```python
from build123d import *

# Parameters (mm, degrees)
SKETCH1_W           = 10
SKETCH1_H           = 8
BOSS_EXTRUDE1_DEPTH = 5
SKETCH2_W           = 9.8
SKETCH2_H           = 1.3
BOSS_EXTRUDE2_DEPTH = 6
SKETCH3_W           = 6.3
SKETCH3_H           = 0.5
BOSS_EXTRUDE3_DEPTH = 2.5
BOSS_EXTRUDE4_START = -6.3
BOSS_EXTRUDE4_DEPTH = 6.3
SKETCH5_W           = 1.2
SKETCH5_H           = 5
CUT_EXTRUDE1_DEPTH  = 14.190905958
SKETCH6_W           = 0.275
SKETCH6_H           = 5
SKETCH6_W_2         = 0.2
CUT_EXTRUDE2_DEPTH  = 3.5
SKETCH7_R           = 1.8
CUT_EXTRUDE3_DEPTH  = 3.5
SKETCH8_W           = 0.11872329
SKETCH8_H           = 1.322916667
CUT_EXTRUDE4_DEPTH  = 3.5


with BuildPart() as part:
    # Sketch1 → Boss-Extrude1 (new body)
    with BuildSketch(Plane(origin=(0, 0, 0), x_dir=(1, 0, 0), z_dir=(0, 1, 0))):
        Rectangle(SKETCH1_W, SKETCH1_H)
    extrude(amount=BOSS_EXTRUDE1_DEPTH)

    # Sketch2 → Boss-Extrude2 (add)
    with BuildSketch(Plane(origin=(0, 0, -4), x_dir=(-1, 0, 0), z_dir=(0, 0, -1))):
        with Locations((0, 0.65)):
            Rectangle(SKETCH2_W, SKETCH2_H)
    extrude(amount=BOSS_EXTRUDE2_DEPTH)

    # Sketch3 → Boss-Extrude3 (add)
    with BuildSketch(Plane.XY.offset(4)):
        with Locations((0, 3.75)):
            Rectangle(SKETCH3_W, SKETCH3_H)
    extrude(amount=BOSS_EXTRUDE3_DEPTH)

    # Sketch4 → Boss-Extrude4 (add)
    with BuildSketch(Plane.ZY.offset(3.15).offset(BOSS_EXTRUDE4_START)):
        with BuildLine():
            Line((7.714456463, 2), (7.714456463, -3))
            Line((7.714456463, -3), (8.214456463, -3))
            Line((8.214456463, -3), (8.214456463, 2))
            ThreePointArc((8.214456463, 2), (7.756212161, 3.342020289), (6.5, 4))
            Line((6.5, 4), (6.5, 3.5))
            ThreePointArc((6.5, 3.5), (7.40002744, 2.98706126), (7.714456463, 2))
        make_face()
    extrude(amount=BOSS_EXTRUDE4_DEPTH)

    # Sketch5 → Cut-Extrude1 (cut, through all)
    with BuildSketch(Plane(origin=(0, 4, 0), x_dir=(1, 0, 0), z_dir=(0, 1, 0))):
        with Locations((-1.2, -6.5)):
            Rectangle(SKETCH5_W, SKETCH5_H)
        with Locations((1.2, -6.5)):
            Rectangle(SKETCH5_W, SKETCH5_H)
    extrude(amount=-CUT_EXTRUDE1_DEPTH, mode=Mode.SUBTRACT)

    # Sketch6 → Cut-Extrude2 (cut)
    with BuildSketch(Plane.XY.offset(8.214456463)):
        with Locations((-3.0125, -0.5)):
            Rectangle(SKETCH6_W, SKETCH6_H)
        with Locations((-1.9375, -0.5)):
            Rectangle(SKETCH6_W, SKETCH6_H)
        with Locations((-0.5, -0.5)):
            Rectangle(SKETCH6_W_2, SKETCH6_H)
        with Locations((0.5, -0.5)):
            Rectangle(SKETCH6_W_2, SKETCH6_H)
        with Locations((1.9375, -0.5)):
            Rectangle(SKETCH6_W, SKETCH6_H)
        with Locations((3.0125, -0.5)):
            Rectangle(SKETCH6_W, SKETCH6_H)
    extrude(amount=-CUT_EXTRUDE2_DEPTH, mode=Mode.SUBTRACT)

    # Sketch7 → Cut-Extrude3 (cut)
    with BuildSketch(Plane(origin=(0, 1.3, 0), x_dir=(1, 0, 0), z_dir=(0, 1, 0))):
        with Locations(Location((0, 8, 0), (0, 0, 270))):
            Circle(SKETCH7_R)
    extrude(amount=-CUT_EXTRUDE3_DEPTH, mode=Mode.SUBTRACT)

    # Sketch8 → Cut-Extrude4 (cut)
    # profile 1 of 7: a face of its own
    with BuildSketch(Plane(origin=(0, 5, 0), x_dir=(1, 0, 0), z_dir=(0, 1, 0))):
        with Locations((-3.24297038, 1.408129396)):
            Rectangle(SKETCH8_W, SKETCH8_H)
    # profile 2 of 7: a face of its own
    with BuildSketch(Plane(origin=(0, 5, 0), x_dir=(1, 0, 0), z_dir=(0, 1, 0))):
        with BuildLine():
            Line((-2.844399333, 2.069587729), (-2.579656995, 2.069587729))
            add(Edge.make_bspline(
                [(-2.579656995, 2.069587729), (-2.561989961, 2.069528921), (-2.5280673, 2.069416003), (-2.479469665, 2.068786385), (-2.435311804, 2.066981792), (-2.395616805, 2.065428845), (-2.360385397, 2.06259707), (-2.329509546, 2.059890516), (-2.303131458, 2.056347495), (-2.287163532, 2.053057052), (-2.279933688, 2.051567229)],
                knots=[0, 0, 0, 0, 1.410062039, 2.707475311, 3.878576406, 4.937260626, 5.877586885, 6.699081471, 7.410979367, 8, 8, 8, 8], degree=3))
            add(Edge.make_bspline(
                [(-2.279933688, 2.051567229), (-2.270254994, 2.049175863), (-2.251104078, 2.044444144), (-2.22353069, 2.034443045), (-2.19725593, 2.022869555), (-2.172388943, 2.009276125), (-2.149054284, 1.993561849), (-2.127011351, 1.975998005), (-2.106160119, 1.956680698), (-2.087343849, 1.935122886), (-2.069602005, 1.91250611), (-2.054638446, 1.88804963), (-2.04173945, 1.862475184), (-2.031469641, 1.835522678), (-2.023200288, 1.807453496), (-2.017369537, 1.778013385), (-2.013872808, 1.747336469), (-2.013516809, 1.726412498), (-2.013336299, 1.715802923)],
                knots=[0, 0, 0, 0, 1.027469482, 2.033020251, 3.019912614, 3.986113645, 4.951240523, 5.91722682, 6.890402269, 7.87763091, 8.8651537, 9.85103654, 10.82876324, 11.815024772, 12.821070561, 13.842952187, 14.906261191, 16, 16, 16, 16], degree=3))
            add(Edge.make_bspline(
                [(-2.013336299, 1.715802923), (-2.013891545, 1.698175964), (-2.014974974, 1.663781201), (-2.025076427, 1.613865332), (-2.041622909, 1.567302704), (-2.064423676, 1.524151945), (-2.093459609, 1.485254172), (-2.128356182, 1.451088732), (-2.169132862, 1.422498646), (-2.207092753, 1.402672734), (-2.240624608, 1.389975415), (-2.268229461, 1.381041434), (-2.298341682, 1.374138846), (-2.330672758, 1.367955106), (-2.365357235, 1.363286459), (-2.402311982, 1.359867062), (-2.441563355, 1.357729966), (-2.468527824, 1.357411708), (-2.482399299, 1.357247985)],
                knots=[0, 0, 0, 0, 1.260483769, 2.459530307, 3.627416485, 4.787058657, 5.939039949, 7.08810263, 8.267026773, 9.491475466, 10.141966685, 10.831826277, 11.566392101, 12.351337768, 13.187381173, 14.07005841, 15.007169909, 16, 16, 16, 16], degree=3))
            Line((-2.482399299, 1.357247985), (-1.996375829, 0.746671062))
            Line((-1.996375829, 0.746671062), (-2.143189898, 0.746671062))
            Line((-2.143189898, 0.746671062), (-2.629213369, 1.357247985))
            Line((-2.629213369, 1.357247985), (-2.725676042, 1.357247985))
            Line((-2.725676042, 1.357247985), (-2.725676042, 0.746671062))
            Line((-2.725676042, 0.746671062), (-2.844399333, 0.746671062))
            Line((-2.844399333, 0.746671062), (-2.844399333, 2.069587729))
        make_face()
        with BuildLine():
            Line((-2.725676042, 1.933903968), (-2.725676042, 1.492931746))
            Line((-2.725676042, 1.492931746), (-2.483459329, 1.491076694))
            add(Edge.make_bspline(
                [(-2.483459329, 1.491076694), (-2.472150266, 1.491071691), (-2.450230083, 1.491061994), (-2.418517629, 1.492571546), (-2.388990087, 1.494288812), (-2.361760398, 1.496915499), (-2.336816398, 1.500300681), (-2.314170554, 1.504535143), (-2.2937859, 1.509468511), (-2.27001175, 1.517104245), (-2.243464014, 1.529201758), (-2.214612539, 1.546802408), (-2.190043203, 1.56894014), (-2.169285559, 1.594254512), (-2.152605685, 1.622087261), (-2.140846069, 1.652104758), (-2.133383896, 1.683549201), (-2.132503761, 1.705161164), (-2.132059589, 1.71606793)],
                knots=[0, 0, 0, 0, 1.146690395, 2.22261258, 3.21895312, 4.145990853, 4.996080663, 5.770904154, 6.481378293, 7.121626537, 8.300444488, 9.431385265, 10.535395872, 11.636531494, 12.74115979, 13.810798291, 14.895190096, 16, 16, 16, 16], degree=3))
            add(Edge.make_bspline(
                [(-2.132059589, 1.71606793), (-2.132513962, 1.726706665), (-2.133414364, 1.747788755), (-2.140765536, 1.778652745), (-2.153196939, 1.807782217), (-2.169949689, 1.835058675), (-2.190360084, 1.859818283), (-2.21429271, 1.881002772), (-2.241093185, 1.898483969), (-2.26614212, 1.909654821), (-2.288531242, 1.916503694), (-2.307970429, 1.921323331), (-2.329935184, 1.925195496), (-2.354532158, 1.928297947), (-2.381656346, 1.930964548), (-2.411444896, 1.932760608), (-2.443700167, 1.933824181), (-2.466056299, 1.933876754), (-2.477629167, 1.933903968)],
                knots=[0, 0, 0, 0, 1.101028733, 2.181837193, 3.264309656, 4.369019818, 5.486613113, 6.575447106, 7.666700264, 8.788928104, 9.402425223, 10.0903467, 10.862060571, 11.710948788, 12.657782767, 13.684531032, 14.801375019, 16, 16, 16, 16], degree=3))
            Line((-2.477629167, 1.933903968), (-2.725676042, 1.933903968))
        make_face(mode=Mode.SUBTRACT)
    # profile 3 of 7: a face of its own
    with BuildSketch(Plane(origin=(0, 5, 0), x_dir=(1, 0, 0), z_dir=(0, 1, 0))):
        Polygon((-1.725008307, 2.069587729), (-1.606285017, 2.069587729), (-1.606285017, 0.882354823), (-1.097470914, 0.882354823), (-1.097470914, 0.746671062), (-1.725008307, 0.746671062), align=None)
    # profile 4 of 7: a face of its own
    with BuildSketch(Plane(origin=(0, 5, 0), x_dir=(1, 0, 0), z_dir=(0, 1, 0))):
        Polygon((-0.944826683, 1.933903968), (-0.944826683, 2.069587729), (-0.24944741, 2.069587729), (-0.80437279, 0.882354823), (-0.26640788, 0.882354823), (-0.26640788, 0.746671062), (-0.995708093, 0.746671062), (-0.440782713, 1.933903968), align=None)
    # profile 5 of 7: a face of its own
    with BuildSketch(Plane(origin=(0, 5, 0), x_dir=(1, 0, 0), z_dir=(0, 1, 0))):
        Polygon((0.608381366, 2.103508669), (0.632497035, 2.103508669), (0.632497035, 1.187643284), (0.785141265, 1.187643284), (0.785141265, 1.051959524), (0.632497035, 1.051959524), (0.632497035, 0.746671062), (0.513773744, 0.746671062), (0.513773744, 1.051959524), (-0.113763649, 1.051959524), align=None)
        Polygon((0.513773744, 1.187643284), (0.513773744, 1.762179208), (0.119442815, 1.187643284), align=None, mode=Mode.SUBTRACT)
    # profile 6 of 7: a face of its own
    with BuildSketch(Plane(origin=(0, 5, 0), x_dir=(1, 0, 0), z_dir=(0, 1, 0))):
        Polygon((1.626009571, 2.103508669), (1.65012524, 2.103508669), (1.65012524, 1.187643284), (1.802769471, 1.187643284), (1.802769471, 1.051959524), (1.65012524, 1.051959524), (1.65012524, 0.746671062), (1.531401949, 0.746671062), (1.531401949, 1.051959524), (0.903864556, 1.051959524), align=None)
        Polygon((1.531401949, 1.187643284), (1.531401949, 1.762179208), (1.13707102, 1.187643284), align=None, mode=Mode.SUBTRACT)
    # profile 7 of 7: a face of its own
    with BuildSketch(Plane(origin=(0, 5, 0), x_dir=(1, 0, 0), z_dir=(0, 1, 0))):
        Polygon((2.040216052, 0.746671062), (2.040216052, 2.069587729), (2.065126742, 2.069587729), (2.939120966, 1.02837387), (2.939120966, 2.069587729), (3.057844257, 2.069587729), (3.057844257, 0.746671062), (3.030813508, 0.746671062), (2.158939342, 1.785499855), (2.158939342, 0.746671062), align=None)
    extrude(amount=-CUT_EXTRUDE4_DEPTH, mode=Mode.SUBTRACT)


solid = part.part
```
Geometry check sheet. Reference: the model listing, model coordinates, mm. A direction names the side the tool comes from. Coordinates: 2 decimals unless noted, no trailing zeros. Loops run counter-clockwise (first coordinate to the right, second up) from the corner with the lowest first, then second, coordinate; pieces in that order, holes last.
Item 1: Sectioned sample at A-A, the plane y = 0.25. Record the boundary of the cut face in (x, z) (3 decimals), then the cut area to 3 significant figures.
Item 2: Sectioned sample at C-C, the plane y = 2.75. Count the separate pieces of the cut face and the enclosed holes in it, then the cut area to 3 significant figures.
Item 3: Thickness scan on line 1 (X direction, y = 0.9, z = -8); line 2 (Y direction, x = 3.75, z = 1.25); line 3 (Z direction, x = -3.5, y = 0.75). Record the ranges inside material, lowest first.
Item 4: Release check for a two-part mould opening along X. For faces 1 (the face through (4.9, 1, -7)), 2 (the face through (2, 4, 5)), 3 (the face through (0.6, 3.7, 6.3)) record: released by +X, released by -X, zero draft, split by the parting line, or undercut.
Item 5: Access from +Z, -Z, +X, -X, +Y, -Y to the whole of each face (thin tool, end or side, straight path). Record for faces 4 (the face through (-1.8, 3.7, 6.3)), 5 (the face through (-2, 3.5, 5)), 6 (the face through (-2, 4, 5)), 7 (the face through (0, 1, -10)).
Item 6: Go/stop test with flat-tipped pins: pin 1 Ø1 at (x, y) = (-2.5, 4) entering from +Z; pin 2 Ø4 at (x, z) = (-2, 1.5) entering from -Y. Record where each tip stops, or that it passes through.
Item 7: Sectioned sample at D-D, the plane z = -2.5. Record the boundary of the cut face in (x, y).
Item 8: Sectioned sample at B-B, the plane z = -8. Record the boundary of the cut face in (x, y).
Check result:
1. outline: (-5, -4) - (-4.9, -4) - (-4.9, -10) - (4.9, -10) - (4.9, -4) - (5, -4) - (5, 4) - (-5, 4) - close; (-2.875, 7.714) - (-2.075, 7.714) - (-2.075, 8.214) - (-2.875, 8.214) - close; (-0.4, 7.714) - (0.4, 7.714) - (0.4, 8.214) - (-0.4, 8.214) - close; (2.075, 7.714) - (2.875, 7.714) - (2.875, 8.214) - (2.075, 8.214) - close; hole circle Ø3.6 at (0, -8)
1. area: 130 mm2
2. separate pieces: 7
2. enclosed holes: 7
2. area: 79.8 mm2
3. line 1: x = -4.9 to -1.8, 1.8 to 4.9
3. line 2: y = 0 to 5
3. line 3: z = -10 to 4
4. face 1: released by +X
4. face 2: zero draft
4. face 3: undercut
5. face 4: +Z, +Y, -Y
5. face 5: +X, -X, -Y
5. face 6: +Z, +X, -X, +Y
5. face 7: -Z, +X, -X, +Y, -Y
6. pin 1: stops at z = 7.6
6. pin 2: stops at y = 0
7. outline: (-5, 0) - (5, 0) - (5, 5) - (-5, 5) - close
8. outline: (-4.9, 0) - (-1.8, 0) - (-1.8, 1.3) - (-4.9, 1.3) - close; (1.8, 0) - (4.9, 0) - (4.9, 1.3) - (1.8, 1.3) - close
